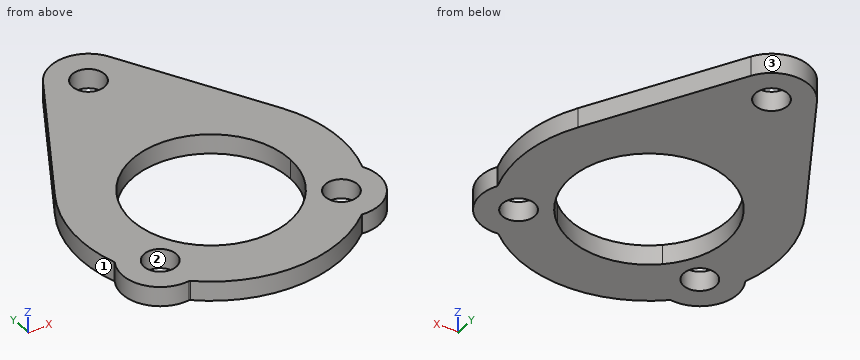
from build123d import *

# Parameters (mm, degrees)
F0_R     = 5.207
F1_DEPTH = 6.35


with BuildPart() as f1:
    # F0 (on Top) → F1 (new body)
    with BuildSketch(Plane.XY):
        with BuildLine():
            Line((36.373199, 20.799049), (10.596841, 65.876522))
            ThreePointArc((10.596841, 65.876522), (0, 72.024), (-10.596841, 65.876522))
            Line((-10.596841, 65.876522), (-36.373199, 20.799049))
            ThreePointArc((-36.373199, 20.799049), (-41.695098, 4.138692), (-39.75222, -13.242772))
            ThreePointArc((-39.75222, -13.242772), (-39.728424, -13.443582), (-39.786109, -13.637394))
            ThreePointArc((-39.786109, -13.637394), (-39.179546, -26.199019), (-27.802439, -31.558475))
            ThreePointArc((-27.802439, -31.558475), (-27.60129, -31.579207), (-27.424803, -31.677913))
            ThreePointArc((-27.424803, -31.677913), (0, -41.9), (27.424803, -31.677913))
            ThreePointArc((27.424803, -31.677913), (27.60129, -31.579207), (27.802439, -31.558475))
            ThreePointArc((27.802439, -31.558475), (39.179546, -26.199019), (39.786109, -13.637394))
            ThreePointArc((39.786109, -13.637394), (39.728424, -13.443582), (39.75222, -13.242772))
            ThreePointArc((39.75222, -13.242772), (41.695098, 4.138692), (36.373199, 20.799049))
        make_face()
        with Locations((-29.0322, -19.413577)):
            Circle(F0_R, mode=Mode.SUBTRACT)
        with Locations((29.0322, -19.413577)):
            Circle(F0_R, mode=Mode.SUBTRACT)
        with BuildLine():
            ThreePointArc((-16.831461, -19.022669), (-10.431704, 23.159006), (25.4, 0))
            ThreePointArc((25.4, 0), (23.159006, -10.431704), (16.831461, -19.022669))
            ThreePointArc((16.831461, -19.022669), (0, -25.4), (-16.831461, -19.022669))
        make_face(mode=Mode.SUBTRACT)
        with Locations((0, 59.817)):
            Circle(F0_R, mode=Mode.SUBTRACT)
    extrude(amount=F1_DEPTH)


solid = f1.part
For this review, take the finished solid that the model builds, in its own axes (mm). Face numbers are marked on the shaded views. Round coordinates to 2 decimals unless told otherwise and drop trailing zeros. Order: outer loops, then holes, each group sorted by start corner. A loop starts at its lowest first (then second) coordinate and runs counter-clockwise, first axis right, second up. Notation, with made-up numbers: M 9,72.25 L 38,72.25 A15 cw 38,86.25 Z; hole C 23.25,24 d5. An arc over 180 degrees is marked long. Use a Markdown table: item, result. Add a question column.
Item 1: Insertion check: pin 1 (8.5 mm diameter, centred on x = 29.03, y = -19.41, fed in from +Z); pin 2 (3 mm diameter, centred on x = -8, z = 1, fed in from +Y). Each pin has a flat end and moves straight along its axis. Give the tip position at first contact, or say it passes through.
Item 2: Add section D-D, the plane x = -15.5. Give the boundary of the cut face in (y, z), then the cut area to 3 significant figures.
Item 3: To check wall thickness, follow line 1 along X through (y, z) = (14.5, 3.5); line 2 along Y through (x, z) = (-20, 0.75); line 3 along Y through (x, z) = (-6, 3). State the ranges of each line that lie inside material, in increasing order.
Item 4: Mouldability with a two-part tool opening along X and no side actions: class the marked faces 1, 2 and 3 as released by +X, released by -X, zero draft, split by the parting line, or undercut.
Item 5: Add section B-B, the plane y = -21.5. Give the boundary of the cut face in (x, z).
Item 6: Add section C-C, the plane y = 13. Give the boundary of the cut face in (x, z), then the cut area to 3 significant figures.
Item 7: Add section A-A, the plane x = 0. Give the boundary of the cut face in (y, z).
Geometry results:
| question | item | result |
|---|---|---|
| 1 | pin 1 | passes through |
| 1 | pin 2 | stops at y = 70.15 |
| 2 | outline | M -38.93,0 L -20.12,0 L -20.12,6.35 L -38.93,6.35 Z; M 20.12,0 L 57.3,0 L 57.3,6.35 L 20.12,6.35 Z |
| 2 | area | 356 mm² |
| 3 | line 1 | x = -39.31 to -20.85, 20.85 to 39.31 |
| 3 | line 2 | y = -36.82 to -15.66, 15.66 to 49.43 |
| 3 | line 3 | y = -41.47 to -24.68, 24.68 to 70.45 |
| 4 | face 1 | released by -X |
| 4 | face 2 | undercut |
| 4 | face 3 | split by the parting line |
| 5 | outline | M -41.06,0 L -33.8,0 L -33.8,6.35 L -41.06,6.35 Z; M -24.26,0 L -13.52,0 L -13.52,6.35 L -24.26,6.35 Z; M 13.52,0 L 24.26,0 L 24.26,6.35 L 13.52,6.35 Z; M 33.8,0 L 41.06,0 L 41.06,6.35 L 33.8,6.35 Z |
| 6 | outline | M -39.83,0 L -21.82,0 L -21.82,6.35 L -39.83,6.35 Z; M 21.82,0 L 39.83,0 L 39.83,6.35 L 21.82,6.35 Z |
| 6 | area | 229 mm² |
| 7 | outline | M -41.9,0 L -25.4,0 L -25.4,6.35 L -41.9,6.35 Z; M 25.4,0 L 54.61,0 L 54.61,6.35 L 25.4,6.35 Z; M 65.02,0 L 72.02,0 L 72.02,6.35 L 65.02,6.35 Z |
